Could you check a few things on this model? Use its own coordinates, in mm. A direction names the side the tool comes from. Coordinates: 2 decimals unless noted, no trailing zeros. Order: outer loops, then holes, each group sorted by start corner. A loop starts at its lowest first (then second) coordinate and runs counter-clockwise, first axis right, second up.
```python
from build123d import *

# Parameters (mm, degrees)
SKETCH1_R           = 37.5
SKETCH1_R_2         = 3.2
BOSS_EXTRUDE1_DEPTH = 5
SKETCH2_R           = 20
BOSS_EXTRUDE2_DEPTH = 68
SKETCH5_R           = 37.5
SKETCH5_R_2         = 3.2
BOSS_EXTRUDE3_DEPTH = 5


with BuildPart() as part:
    # Sketch1 → Boss-Extrude1 (new body)
    with BuildSketch(Plane(origin=(0, 0, 0), x_dir=(1, 0, 0), z_dir=(0, 1, 0))):
        Circle(SKETCH1_R)
        with Locations((0, 31)):
            Circle(SKETCH1_R_2, mode=Mode.SUBTRACT)
        with Locations((26.846787517, 15.5)):
            Circle(SKETCH1_R_2, mode=Mode.SUBTRACT)
        with Locations((26.846787517, -15.5)):
            Circle(SKETCH1_R_2, mode=Mode.SUBTRACT)
        with Locations((0, -31)):
            Circle(SKETCH1_R_2, mode=Mode.SUBTRACT)
        with Locations((-26.846787517, -15.5)):
            Circle(SKETCH1_R_2, mode=Mode.SUBTRACT)
        with Locations((-26.846787517, 15.5)):
            Circle(SKETCH1_R_2, mode=Mode.SUBTRACT)
    extrude(amount=BOSS_EXTRUDE1_DEPTH)

    # Sketch2 → Boss-Extrude2 (add)
    with BuildSketch(Plane(origin=(0, 5, 0), x_dir=(1, 0, 0), z_dir=(0, 1, 0))):
        Circle(SKETCH2_R)
    extrude(amount=BOSS_EXTRUDE2_DEPTH)

    # Sketch5 → Boss-Extrude3 (add)
    with BuildSketch(Plane(origin=(0, 73, 0), x_dir=(1, 0, 0), z_dir=(0, 1, 0))):
        with Locations((0.421553843, 0.250555935)):
            Circle(SKETCH5_R)
        with Locations((0.421553843, 31.250555935)):
            Circle(SKETCH5_R_2, mode=Mode.SUBTRACT)
        with Locations((27.268341361, 15.750555935)):
            Circle(SKETCH5_R_2, mode=Mode.SUBTRACT)
        with Locations((27.268341361, -15.249444065)):
            Circle(SKETCH5_R_2, mode=Mode.SUBTRACT)
        with Locations((0.421553843, -30.749444065)):
            Circle(SKETCH5_R_2, mode=Mode.SUBTRACT)
        with Locations((-26.425233674, -15.249444065)):
            Circle(SKETCH5_R_2, mode=Mode.SUBTRACT)
        with Locations((-26.425233674, 15.750555935)):
            Circle(SKETCH5_R_2, mode=Mode.SUBTRACT)
    extrude(amount=BOSS_EXTRUDE3_DEPTH)


solid = part.part
```
Item 1: Which directions (+Z, -Z, +X, -X, +Y, -Y) give clear straight access to the entire face, cutting with the end or side of a thin tool? Please do faces 1 (the face through (24.31, 2.46, -13.55)), 2 (the face through (-0.272, 75.465, -28.127)), 3 (the face through (-1, 0, -1)), 4 (the face through (16, 5, 16)).
Item 2: For pin 1 Ø6 at (y, z) = (11, -15) entering from -X; pin 2 Ø12 at (x, y) = (-2.5, 10.5) entering from -Z; pin 3 Ø2 at (x, y) = (17.5, 44) entering from +Z, each with a flat end and sliding along its axis, tell me the tip position at first contact or that it passes through.
Item 3: I need wall thicknesses on line 1 (Z direction, x = 0, y = 2); line 2 (Y direction, x = 29, z = 10.5); line 3 (X direction, y = 1.15, z = 15.5). Which ranges of each line are inside material? Lowest first, please.
Item 4: Suppose I cut it at A-A (x = 0). List the corners of the cut face in (y, z) for me, and give its area (3 significant figures).
Item 5: Thinking about a two-plate mould opening in X: for faces 5 (the face through (-4.88, 2.46, -37.18)), 6 (the face through (24.31, 2.46, 17.45)), 7 (the face through (0, 78, -1)), which applies, +X half, -X half, draft (parallel to the pull), parting line (faces both ways), or undercut?
Item 6: Suppose I cut it at D-D (x = 10). List the corners of the cut face in (y, z) for me.
Item 7: Suppose I cut it at B-B (x = 33). List the corners of the cut face in (y, z) for me, and give its area (3 significant figures).
Item 8: Suppose I cut it at C-C (y = 29). List the corners of the cut face in (x, z) for me, and give its area (3 significant figures).
Geometry results:
1. face 1: -Y
1. face 2: +Y
1. face 3: +Z, -Z, +X, -X, -Y
1. face 4: none
2. pin 1: stops at x = -16
2. pin 2: stops at z = -37.5
2. pin 3: stops at z = 11.3
3. line 1: z = -37.5 to -34.2, -27.8 to 27.8, 34.2 to 37.5
3. line 2: y = 0 to 5, 73 to 78
3. line 3: x = -34.15 to -30.05, -23.65 to 23.65, 30.05 to 34.15
4. outline: (0, -37.5) - (5, -37.5) - (5, -34.2) - (0, -34.2) - close; (0, -27.8) - (5, -27.8) - (5, -20) - (73, -20) - (73, -28.08) - (78, -28.08) - (78, 27.58) - (73, 27.58) - (73, 20) - (5, 20) - (5, 27.8) - (0, 27.8) - close; (0, 34.2) - (5, 34.2) - (5, 37.5) - (0, 37.5) - close; (73, -37.75) - (78, -37.75) - (78, -34.42) - (73, -34.42) - close; (73, 33.92) - (78, 33.92) - (78, 37.25) - (73, 37.25) - close
4. area: 3,340 mm2
5. face 5: parting line
5. face 6: undercut
5. face 7: draft
6. outline: (0, -36.14) - (5, -36.14) - (5, -17.32) - (73, -17.32) - (73, -36.51) - (78, -36.51) - (78, 36.01) - (73, 36.01) - (73, 17.32) - (5, 17.32) - (5, 36.14) - (0, 36.14) - close
7. outline: (0, -17.81) - (5, -17.81) - (5, 17.81) - (0, 17.81) - close; (73, -18.82) - (78, -18.82) - (78, 18.32) - (73, 18.32) - close
7. area: 364 mm2
8. outline: circle Ø40 at (0, 0)
8. area: 1,260 mm2
